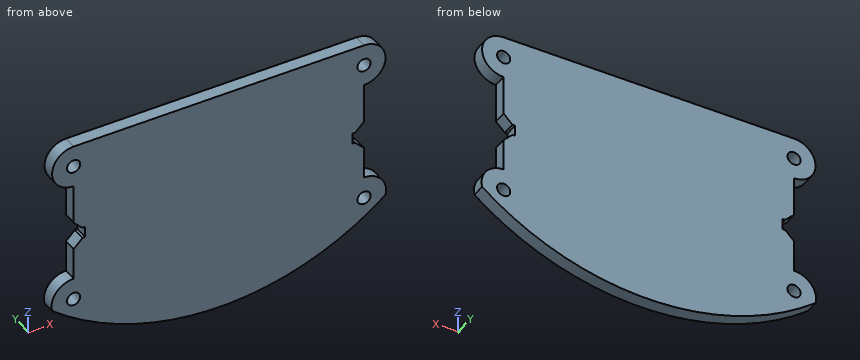
```python
from build123d import *

# Parameters (mm, degrees)
CROQUIS1_R              = 1.5
SALIENTE_EXTRUIR1_DEPTH = 3


with BuildPart() as part:
    # Croquis1 → Saliente-Extruir1 (new body)
    with BuildSketch(Plane(origin=(0, 0, 0), x_dir=(1, 0, 0), z_dir=(0, 1, 0))):
        with BuildLine():
            Line((-32.89, -7.25), (-32.89, 0.008962831))
            Line((-32.89, 0.008962831), (-32.892040435, 0.008962415))
            ThreePointArc((-32.892040435, 0.008962415), (-36.801169554, 1.891477927), (-37.766700191, 6.121478601))
            ThreePointArc((-37.766700191, 6.121478601), (0, 19.498776441), (37.766700191, 6.121478601))
            ThreePointArc((37.766700191, 6.121478601), (36.801169554, 1.891477927), (32.892040435, 0.008962415))
            Line((32.892040435, 0.008962415), (32.89, 0.008962831))
            Line((32.89, 0.008962831), (32.89, -7.25))
            Line((32.89, -7.25), (30.89, -9.25))
            Line((30.89, -9.25), (30.29, -9.25))
            Line((30.29, -9.25), (30.29, -11.749506691))
            Line((30.29, -11.749506691), (30.89, -11.749506691))
            Line((30.89, -11.749506691), (32.89, -13.749506691))
            Line((32.89, -13.749506691), (32.89, -22.746599618))
            ThreePointArc((32.89, -22.746599618), (37.766700191, -27.623299809), (32.89, -32.5))
            Line((32.89, -32.5), (-32.89, -32.5))
            ThreePointArc((-32.89, -32.5), (-37.766700191, -27.623299809), (-32.89, -22.746599618))
            Line((-32.89, -22.746599618), (-32.89, -13.749506691))
            Line((-32.89, -13.749506691), (-30.89, -11.749506691))
            Line((-30.89, -11.749506691), (-30.29, -11.749506691))
            Line((-30.29, -11.749506691), (-30.29, -9.25))
            Line((-30.29, -9.25), (-30.89, -9.25))
            Line((-30.89, -9.25), (-32.89, -7.25))
        make_face()
        with Locations(Location((-32.892040435, 5.008962415, 0), (0, 0, 270))):
            Circle(CROQUIS1_R, mode=Mode.SUBTRACT)
        with Locations(Location((32.89, 5.008962415, 0), (0, 0, 270))):
            Circle(CROQUIS1_R, mode=Mode.SUBTRACT)
        with Locations(Location((-32.89, -27.623299809, 0), (0, 0, 270))):
            Circle(CROQUIS1_R, mode=Mode.SUBTRACT)
        with Locations(Location((32.89, -27.623299809, 0), (0, 0, 270))):
            Circle(CROQUIS1_R, mode=Mode.SUBTRACT)
    extrude(amount=SALIENTE_EXTRUIR1_DEPTH)


solid = part.part
```
For this review, take the finished solid that the model builds, in its own axes (mm). Coordinates: 2 decimals unless noted, no trailing zeros. Loops run counter-clockwise (first coordinate to the right, second up) from the corner with the lowest first, then second, coordinate; pieces in that order, holes last.
1. Add section A-A, the plane y = 2.4. Count the separate pieces of the cut face and the enclosed holes in it, then the cut area to 3 significant figures.
2. Add section C-C, the plane x = 13. Give the boundary of the cut face in (y, z), then the cut area to 3 significant figures.
3. Insertion check: P1, Ø0.9, axis at y = 1, z = 20, coming from the +X side; P2, Ø0.7, axis at y = 2, z = 11, coming from the +X side; P3, Ø1.5, axis at y = 1.5, z = 18.5, coming from the -X side. Each pin has a flat end and moves straight along its axis. Give the tip position at first contact, or say it passes through.
4. For line 1 (X direction, y = 0.95, z = 28); line 2 (X direction, y = 2.45, z = 19); line 3 (Z direction, x = 33, y = 1.3), list the stretches that pass through material, from the lowest coordinate up.
5. Add section B-B, the plane z = 16.5. Give the boundary of the cut face in (x, y), then the cut area to 3 significant figures.
Result:
1. separate pieces: 1
1. enclosed holes: 4
1. area: 3,310 mm2
2. outline: (0, -18.07) - (3, -18.07) - (3, 32.5) - (0, 32.5) - close
2. area: 152 mm2
3. P1: stops at x = 32.89
3. P2: stops at x = 30.29
3. P3: stops at x = -32.89
4. line 1: x = -37.75 to -34.34, -31.44 to 31.44, 34.34 to 37.75
4. line 2: x = -32.89 to 32.89
4. line 3: z = -9.61 to -6.5, -3.51 to -0.01, 22.75 to 26.13, 29.12 to 32.5
5. outline: (-32.89, 0) - (32.89, 0) - (32.89, 3) - (-32.89, 3) - close
5. area: 197 mm2
